For this review, take the finished solid that the model builds, in its own axes (mm). A direction names the side the tool comes from. Coordinates: 2 decimals unless noted, no trailing zeros. Order: outer loops, then holes, each group sorted by start corner. A loop starts at its lowest first (then second) coordinate and runs counter-clockwise, first axis right, second up. Notation, with made-up numbers: (52, 24.5) -> (109, 24.5) arc R13 ccw to (109, 29.5) -> close; hole circle Ø11 at (11.5, -28.5). An arc over 180 degrees is marked (long way). Answer as a JSON object with one key per item and string values. Group by question number.
1) Add section B-B, the plane x = -9. Write out the cut boundary in (y, z).
2) Machinability: for faces 4 (the flat face through (-11.5, -3, 0.9)), 5 (the flat face through (-1.4, 2.6, -1.13)), 6 (the flat face through (14.43, 3, 2)), which of the approach directions +Z, -Z, +X, -X, +Y, -Y give a long, thin tool a straight path to every point of the face, cutting with its end or side? Answer none if there is none.
3) Add section D-D, the plane z = -0.5. Write out the cut boundary in (x, y).
4) Add section C-C, the plane x = -12.5. Write out the cut boundary in (y, z), then the cut area to 3 significant figures.
5) Wall thickness on L1, parallel to Z at x = -4, y = 4; L2, parallel to Z at x = -3.5, y = 0.75; L3, parallel to X at y = 0.25, z = 3: over which ranges is each line inside the solid? List them lowest first.
6) Add section A-A, the plane y = -1.5. Count the separate pieces of the cut face and the enclosed holes in it, then the cut area to 3 significant figures.
7) Draft analysis for pull direction Z (two halves, no side actions). For faces 1 (the flat face through (-14.775, 3.676, 2.19)), 2 (the flat face through (-5.96, 2.6, -1.6)), 3 (the flat face through (0, 5.06, -2)), state which applies: +Z half, -Z half, draft (parallel to the pull), parting line (faces both ways), or undercut.
8) For pin 1 (2 mm diameter, centred on x = -9.5, z = -1.5, fed in from -Y); pin 2 (1.5 mm diameter, centred on x = 4.5, y = 0.5, fed in from +Z), all flat-tipped, find the tip position at first contact; note any pin that passes through.
from build123d import *

# Parameters (mm, degrees)
BOSS_EXTRUDE1_DEPTH = 15.11
BOSS_EXTRUDE2_DEPTH = 0.68
SKETCH3_W           = 1
SKETCH3_H           = 1
CUT_EXTRUDE1_DEPTH  = 6.06
SKETCH4_R           = 0.5
BOSS_EXTRUDE3_DEPTH = 3
LPATTERN1_COUNT     = 12
LPATTERN1_PITCH     = 2.54


with BuildPart() as part:
    # Sketch1 → Boss-Extrude1 (new body, symmetric)
    with BuildSketch(Plane(origin=(0, 0, 0), x_dir=(0, 0, -1), z_dir=(1, 0, 0))):
        Polygon((-2.77, 0), (3.23, 0), (3.23, 5.06), (0, 5.06), (0, 1.83), (-2.77, 1.83), align=None)
    extrude(amount=BOSS_EXTRUDE1_DEPTH, both=True)

    # Sketch2 → Boss-Extrude2 (add)
    with BuildSketch(Plane(origin=(15.11, 0, 0), x_dir=(0, 0, -1), z_dir=(1, 0, 0))):
        Polygon((-4.32, 0), (-4.32, 2.33), (0, 5.06), (0, 0), align=None)
    boss_extrude2 = extrude(amount=-BOSS_EXTRUDE2_DEPTH)

    # Mirror1: Boss-Extrude2 across plane
    add(boss_extrude2.mirror(Plane(origin=(0, 0, 0), x_dir=(0, 0, 1), z_dir=(1, 0, 0))))

    # Sketch3 → Cut-Extrude1 (cut, through all)
    with BuildSketch(Plane(origin=(0, 5.06, 0), x_dir=(1, 0, 0), z_dir=(0, 1, 0))):
        with Locations((13.86, 1.63)):
            Rectangle(SKETCH3_W, SKETCH3_H)
    cut_extrude1 = extrude(amount=-CUT_EXTRUDE1_DEPTH, mode=Mode.SUBTRACT)

    # Sketch4 → Boss-Extrude3 (add)
    with BuildSketch(Plane(origin=(0, 0, 0), x_dir=(1, 0, 0), z_dir=(0, 1, 0))):
        with Locations((13.86, -0.91)):
            Circle(SKETCH4_R)
    boss_extrude3 = extrude(amount=-BOSS_EXTRUDE3_DEPTH)

    # LPattern1: Cut-Extrude1, Boss-Extrude3 ×12
    with Locations(*[(-i * LPATTERN1_PITCH, 0, 0) for i in range(1, LPATTERN1_COUNT)]):
        add(cut_extrude1, mode=Mode.SUBTRACT)
        add(boss_extrude3)


solid = part.part
Output values:
{
 "1": {"outline": "(-3, 0.41) -> (0, 0.41) -> (0, -1.13) -> (5.06, -1.13) -> (5.06, 0) -> (1.83, 0) -> (1.83, 2.77) -> (0, 2.77) -> (0, 1.41) -> (-3, 1.41) -> close; (0, -3.23) -> (5.06, -3.23) -> (5.06, -2.13) -> (0, -2.13) -> close"},
 "2": {"face 4": "+Z, -Z, +X, -X, -Y", "face 5": "+Y, -Y", "face 6": "+Z, +Y"},
 "3": {"outline": "(-15.11, 0) -> (15.11, 0) -> (15.11, 5.06) -> (-15.11, 5.06) -> close"},
 "4": {"outline": "(0, -3.23) -> (5.06, -3.23) -> (5.06, 0) -> (1.83, 0) -> (1.83, 2.77) -> (0, 2.77) -> close", "area": "21.4 mm²"},
 "5": {"L1": "z = -3.23 to -2.13, -1.13 to 0", "L2": "z = -3.23 to -2.13, -1.13 to 2.77", "L3": "x = -15.11 to -14.43, 14.43 to 15.11"},
 "6": {"separate pieces": "12", "enclosed holes": "0", "area": "9.42 mm²"},
 "7": {"face 1": "+Z half", "face 2": "undercut", "face 3": "draft"},
 "8": {"pin 1": "stops at y = 0", "pin 2": "stops at z = 2.77"}
}
